Source: CAD feature listing. Evaluate the final solid. Frame: model axes, mm. Give positions to 0.01 mm unless a question says otherwise; leave off trailing zeros. Order: outer loops, then holes, each group sorted by start corner. A loop starts at its lowest first (then second) coordinate and runs counter-clockwise, first axis right, second up. Notation, with made-up numbers: M 51.5,62 L 104.5,62 A13 cw 104.5,79 Z; hole C 33.5,84 d6. An arc over 180 degrees is marked long. Answer as a JSON object with one key per item and string values. Group by question number.
1. Section query A-A (z = 6). Output: boundary loops of the cut face in (x, y), plus the area to 3 significant figures.
2. Section query B-B (y = 0.45). Output: boundary loops of the cut face in (x, z), plus the area to 3 significant figures.
3. Material intervals for L1, parallel to Z at x = 2, y = 0.25; L2, parallel to Z at x = -2, y = 0.4; L3, parallel to X at y = 0.3, z = -6, sorted ascending. Write a range as [from, to].
4. Pull-direction query (X, two-part tool) for faces 1 (the cylindrical face through (-3.465, 0.986, -7.449)), 2 (the cylindrical face through (2.668, 0.444, -3.21)), 3 (the cylindrical face through (3.465, 0.986, 7.449)), 4 (the cylindrical face through (2.647, 0.444, 3.268)); classes: +X half, -X half, draft (parallel to the pull), parting line (faces both ways), or undercut.
5. Section query D-D (z = 3). Output: boundary loops of the cut face in (x, y).
6. Section query C-C (x = -2). Output: boundary loops of the cut face in (y, z).
7. Pin query (flat end, axial travel): P1, Ø1.7, axis at x = -2, z = -6, coming from the -Y side. Return the tip coordinate at first contact, or that it passes through.
from build123d import *

# Parameters (mm, degrees)
SKETCH1_R                                       = 0.95
SKETCH1_R_2                                     = 0.7
BOSS_EXTRUDE1_DEPTH                             = 2
CSK_FOR_M2_FLAT_HEAD_MACHINE_SCREW1_D           = 1.4
CSK_FOR_M2_FLAT_HEAD_MACHINE_SCREW1_CSINK_D     = 3.6
CSK_FOR_M2_FLAT_HEAD_MACHINE_SCREW1_CSINK_ANGLE = 90


with BuildPart() as part:
    # Sketch1 → Boss-Extrude1 (new body)
    with BuildSketch(Plane(origin=(0, 0, 0), x_dir=(1, 0, 0), z_dir=(0, 1, 0))):
        with BuildLine():
            Line((-2.75, 7.75), (2.75, 7.75))
            ThreePointArc((2.75, 7.75), (3.457106781, 7.457106781), (3.75, 6.75))
            Line((3.75, 6.75), (3.75, -6.75))
            ThreePointArc((3.75, -6.75), (3.457106781, -7.457106781), (2.75, -7.75))
            Line((2.75, -7.75), (-2.75, -7.75))
            ThreePointArc((-2.75, -7.75), (-3.457106781, -7.457106781), (-3.75, -6.75))
            Line((-3.75, -6.75), (-3.75, 6.75))
            ThreePointArc((-3.75, 6.75), (-3.457106781, 7.457106781), (-2.75, 7.75))
        make_face()
        with Locations((-2, 6)):
            Circle(SKETCH1_R, mode=Mode.SUBTRACT)
        with Locations((-2, -6)):
            Circle(SKETCH1_R, mode=Mode.SUBTRACT)
        with Locations((2, 3)):
            Circle(SKETCH1_R_2, mode=Mode.SUBTRACT)
        with Locations((2, -3)):
            Circle(SKETCH1_R_2, mode=Mode.SUBTRACT)
    extrude(amount=BOSS_EXTRUDE1_DEPTH)

    # CSK for M2 Flat Head Machine Screw1 (through all)
    with Locations(Plane(origin=(-2, 2, 6), x_dir=(0, 0, 1), z_dir=(0, 1, 0))):
        with Locations((0, 0), (-12, 0), (-3, 4), (-9, 4)):
            CounterSinkHole(CSK_FOR_M2_FLAT_HEAD_MACHINE_SCREW1_D / 2, CSK_FOR_M2_FLAT_HEAD_MACHINE_SCREW1_CSINK_D / 2, counter_sink_angle=CSK_FOR_M2_FLAT_HEAD_MACHINE_SCREW1_CSINK_ANGLE)


solid = part.part
Answer sheet:
{
 "1": {"outline": "M -3.75,0 L -2.95,0 L -2.95,1.15 L -3.75,1.95 Z; M -1.05,0 L 3.75,0 L 3.75,2 L -0.2,2 L -1.05,1.15 Z", "area": "10.5 mm^2"},
 "2": {"outline": "M -3.75,-6.75 A1 ccw -2.75,-7.75 L 2.75,-7.75 A1 ccw 3.75,-6.75 L 3.75,6.75 A1 ccw 2.75,7.75 L -2.75,7.75 A1 ccw -3.75,6.75 Z; hole C -2,-6 d1.9; hole C -2,6 d1.9; hole C 2,-3 d1.4; hole C 2,3 d1.4", "area": "107 mm^2"},
 "3": {"L1": "[-7.75, -3.7], [-2.3, 2.3], [3.7, 7.75]", "L2": "[-7.75, -6.95], [-5.05, 5.05], [6.95, 7.75]", "L3": "[-3.75, -2.95], [-1.05, 3.75]"},
 "4": {"face 1": "-X half", "face 2": "undercut", "face 3": "+X half", "face 4": "undercut"},
 "5": {"outline": "M -3.75,0 L 1.3,0 L 1.3,0.9 L 0.2,2 L -3.75,2 Z; M 2.7,0 L 3.75,0 L 3.75,1.95 L 2.7,0.9 Z"},
 "6": {"outline": "M 0,-7.75 L 1.95,-7.75 L 1.15,-6.95 L 0,-6.95 Z; M 0,-5.05 L 1.15,-5.05 L 2,-4.2 L 2,4.2 L 1.15,5.05 L 0,5.05 Z; M 0,6.95 L 1.15,6.95 L 1.95,7.75 L 0,7.75 Z"},
 "7": {"P1": "through"}
}
